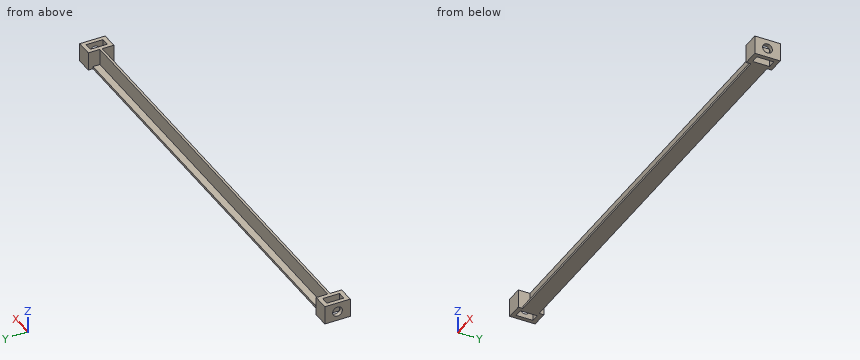
Autodesk Inventor part; units mm, degrees
ref_plane "XZ Plane" through (0, 0, 0) normal (0, 1, 0) x (-1, 0, 0)
ref_plane "XY Plane" through (0, 0, 0) normal (0, 0, 1) x (1, 0, 0)
sketch "Sketch1" plane through (0, 0, 0) normal (0, 0, 1) x (1, 0, 0)
  line L0 (0, 0) -> (200, 0)
  line L1 (200, 0) -> (200, 7)
  line L2 (200, 7) -> (0, 7)
  line L3 (0, 7) -> (0, 0)
  dimension "d0" = 200
  dimension "d1" = 7
extrude "Extrusion1" add sketch "Sketch1" along normal blind 1.5
sketch "Sketch2" plane through (0, 0, 1.5) normal (0, 0, 1) x (1, 0, 0)
  line L0 (200, 7) -> (0, 7)
  line L1 (0, 7) -> (0, 0)
  line L2 (0, 4.25) -> (200, 4.25)
  line L3 (200, 4.25) -> (200, 2.75)
  line L4 (200, 2.75) -> (0, 2.75)
  line L5 (0, 2.75) -> (0, 4.25)
  dimension "d4" = 200
  dimension "d5" = 1.5
  dimension "d6" = 2.75
extrude "Extrusion2" add sketch "Sketch2" along normal blind 6.5
sketch "Sketch3" plane through (0, 0, 0) normal (0, 0, -1) x (-1, 0, 0)
  line L0 (-200, 7) -> (0, 7)
  line L1 (-200, 9) -> (-193, 9)
  line L2 (-193, 9) -> (-193, -2)
  line L3 (-193, -2) -> (-200, -2)
  line L4 (-200, -2) -> (-200, 9)
  dimension "d9" = 7
  dimension "d10" = 11
  dimension "d11" = 2
extrude "Extrusion3" add sketch "Sketch3" against normal up to surface (8 mm away)
sketch "Sketch4" plane through (0, 0, 0) normal (0, 0, -1) x (-1, 0, 0)
  line L0 (-200, 9) -> (-193, 9)
  line L1 (-200, -2) -> (-200, 9)
  line L2 (-193, -2) -> (-200, -2)
  line L3 (-198.25, 7.15) -> (-194.75, 7.15)
  line L4 (-194.75, 7.15) -> (-194.75, -0.15)
  line L5 (-194.75, -0.15) -> (-198.25, -0.15)
  line L6 (-198.25, -0.15) -> (-198.25, 7.15)
  dimension "d14" = 3.5
  dimension "d15" = 7.3
  dimension "d16" = 1.85
  dimension "d17" = 1.85
  dimension "d18" = 1.75
extrude "Extrusion4" cut sketch "Sketch4" against normal blind 8
sketch "Sketch5" plane through (200, -2, 0) normal (1, 0, 0) x (0, 0, -1)
  circle A0 centre (-4, 5.5) radius 2.1
  point P0 (0, 2)
  dimension "d21" = 4.2
ref_plane "Work Plane1" through (100, 0, 0) normal (1, 0, 0) x (0, 1, 0)
extrude "Extrusion5" cut sketch "Sketch5" against normal up to surface (7 mm away)
mirror "Mirror1" about plane through (100, 0, 0) normal (1, 0, 0) of "Extrusion3"
mirror "Mirror2" about plane through (100, 0, 0) normal (1, 0, 0) of "Extrusion5", "Extrusion4"
sketch "Sketch6" plane through (0, 0, 1.5) normal (0, 0, 1) x (1, 0, 0)
  line L0 (7, 7) -> (7, 4.25)
  line L1 (7, 4.25) -> (193, 4.25)
  line L2 (193, 4.25) -> (193, 7)
  line L3 (193, 7) -> (7, 7)
  point P0 (0, 0)
extrude "Extrusion6" cut sketch "Sketch6" against normal blind 0.5
sketch "Sketch7" plane through (0, 0, 1.5) normal (0, 0, 1) x (1, 0, 0)
  line L0 (7, 2.75) -> (7, 0)
  line L1 (7, 0) -> (193, 0)
  line L2 (193, 0) -> (193, 2.75)
  line L3 (193, 2.75) -> (7, 2.75)
  point P0 (0, 0)
extrude "Extrusion7" cut sketch "Sketch7" against normal blind 0.5
sketch "Sketch8" plane through (193, 4.25, 5.9615) normal (0, 1, 0) x (1, 0, 0)
  line L0 (-186, 4.9615) -> (-186, 3.923)
  line L1 (-186, 3.923) -> (-186, 0)
  line L2 (-186, 0) -> (-186, -2.0385)
  line L3 (0, -2.0385) -> (-186, -2.0385)
  line L4 (0, -2.0385) -> (0, 0)
  line L5 (0, 0) -> (0, 3.923)
  line L6 (0, 3.923) -> (0, 4.9615)
  line L7 (0, 4.9615) -> (-186, 4.9615)
  point P0 (-193, 5.9615)
extrude "Extrusion8" cut sketch "Sketch8" against normal blind 0.25
sketch "Sketch9" plane through (193, 2.75, 2.0385) normal (0, -1, 0) x (1, 0, 0)
  line L0 (-186, 5.9615) -> (-186, 3.923)
  line L1 (-186, 3.923) -> (-186, 0)
  line L2 (-186, 0) -> (-186, -1.0385)
  line L3 (-186, -1.0385) -> (0, -1.0385)
  line L4 (0, -1.0385) -> (0, 0)
  line L5 (0, 0) -> (0, 3.923)
  line L6 (0, 3.923) -> (0, 5.9615)
  line L7 (-186, 5.9615) -> (0, 5.9615)
  point P0 (-193, -2.0385)
extrude "Extrusion9" cut sketch "Sketch9" against normal blind 0.25
sketch "Sketch10" plane through (194.75, -0.15, 0) normal (1, 0, 0) x (0, 0, -1)
  circle A0 centre (-4, 3.65) radius 2.1
  point P0 (0, 0.15)
extrude "Extrusion10" add sketch "Sketch10" against normal up to surface (1.75 mm away)
mirror "Mirror3" about plane through (100, 0, 0) normal (1, 0, 0) of "Extrusion10"
properties part number "Axle"
Design review of the part built by this model. Coordinates are the model's own, in mm. Round coordinates to 2 decimals unless told otherwise and drop trailing zeros. Write each loop counter-clockwise with the first axis right and the second up, starting at its lowest first coordinate (ties: lowest second). Pieces come first, ordered by that corner, then holes. Notation, with made-up numbers: (69, 61) - (98, 61) arc R25 cw to (98, 94) - close; hole circle Ø10 at (65.5, 49.25). An arc over 180 degrees is marked (long way). Return JSON: item names as keys, results as strings. Group by question number.
Item 1: For probe 1 along X at (y, z) = (0, 2.25); probe 2 along X at (y, z) = (3.5, 6.25); probe 3 along Y at (x, z) = (1.1, 4), list the stretches that pass through material, from the lowest coordinate up. Write a range as [from, to].
Item 2: Insertion check: P1, Ø3, axis at x = 123, z = 4.5, coming from the +Y side; P2, Ø0.9, axis at x = 114, y = 5, coming from the +Z side; P3, Ø3.5, axis at y = 3.5, z = 4, coming from the -X side. Each pin has a flat end and moves straight along its axis. Give the tip position at first contact, or say it passes through.
Item 3: We need section A-A on z = 4. Write out the cut boundary in (x, y), and give its area (3 significant figures).
Item 4: We need section B-B on x = 171. Write out the cut boundary in (y, z), and give its area (3 significant figures).
Model answer:
{
 "1": {"probe 1": "x = [0, 1.75], [5.25, 7], [193, 194.75], [198.25, 200]", "probe 2": "x = [0, 1.75], [5.25, 194.75], [198.25, 200]", "probe 3": "y = [-2, 1.4], [5.6, 9]"},
 "2": {"P1": "stops at y = 4", "P2": "stops at z = 1", "P3": "stops at x = 5.25"},
 "3": {"outline": "(0, -2) - (7, -2) - (7, 3) - (193, 3) - (193, -2) - (200, -2) - (200, 1.4) - (198.25, 1.4) - (198.25, -0.15) - (194.75, -0.15) - (194.75, 7.15) - (198.25, 7.15) - (198.25, 5.6) - (200, 5.6) - (200, 9) - (193, 9) - (193, 4) - (7, 4) - (7, 9) - (0, 9) - (0, 5.6) - (1.75, 5.6) - (1.75, 7.15) - (5.25, 7.15) - (5.25, -0.15) - (1.75, -0.15) - (1.75, 1.4) - (0, 1.4) - close", "area": "274 mm²"},
 "4": {"outline": "(0, 0) - (7, 0) - (7, 1) - (4, 1) - (4, 8) - (3, 8) - (3, 1) - (0, 1) - close", "area": "14.0 mm²"}
}
